For this review, use the dimensioned drawing (mm, ordinates from the lowest corner) and the shaded views. A direction names the side the tool comes from. Coordinates: 2 decimals unless noted, no trailing zeros. Loops run counter-clockwise (first coordinate to the right, second up) from the corner with the lowest first, then second, coordinate; pieces in that order, holes last. Notation, with made-up numbers: (15.25, 73.25) - (47.25, 73.25) arc R21 ccw to (47.25, 81.25) - close; hole circle Ø1 at (-30.5, -13). An arc over 180 degrees is marked (long way). Use a Markdown table: item, result. Add a question column.
1) The part is to be moulded in two halves that separate along Y. For the marked faces 1, 2 and 3, say which applies: pulls with the +Y half, pulls with the -Y half, needs draft (parallel to the pull), parting line crosses it, or undercut.
2) Add section C-C, the plane y = 45. Give the boundary of the cut face in (x, z), and give its area (3 significant figures).
3) Add section A-A, the plane z = 18. Give the boundary of the cut face in (x, y), and give its area (3 significant figures).
4) Add section D-D, the plane x = 43.5. Give the boundary of the cut face in (y, z), and give its area (3 significant figures).
5) For the marked faces 4 and 5, list the 3-axis set-ups (+Z, -Z, +X, -X, +Y, -Y) from which the entire face can be reached by the end or side of a thin tool; tool diameter is ignored.
6) Add section B-B, the plane x = 130. Give the boundary of the cut face in (y, z).
7) Clearance check with flat-ended pins moving along their axes: pin 1 (19 mm diameter, centred on x = 44.5, y = 32, fed in from -Z); pin 2 (6 mm diameter, centred on x = 19.5, z = 35, fed in from +Y). State where each tip first meets the part, or that it passes through.
8) To check wall thickness, follow L1, parallel to Y at x = 86.5, z = 7; L2, parallel to Z at x = 14.5, y = 57; L3, parallel to Y at x = 130, z = 35. State the ranges of each line that lie inside material, in increasing order. Write a range as [from, to].
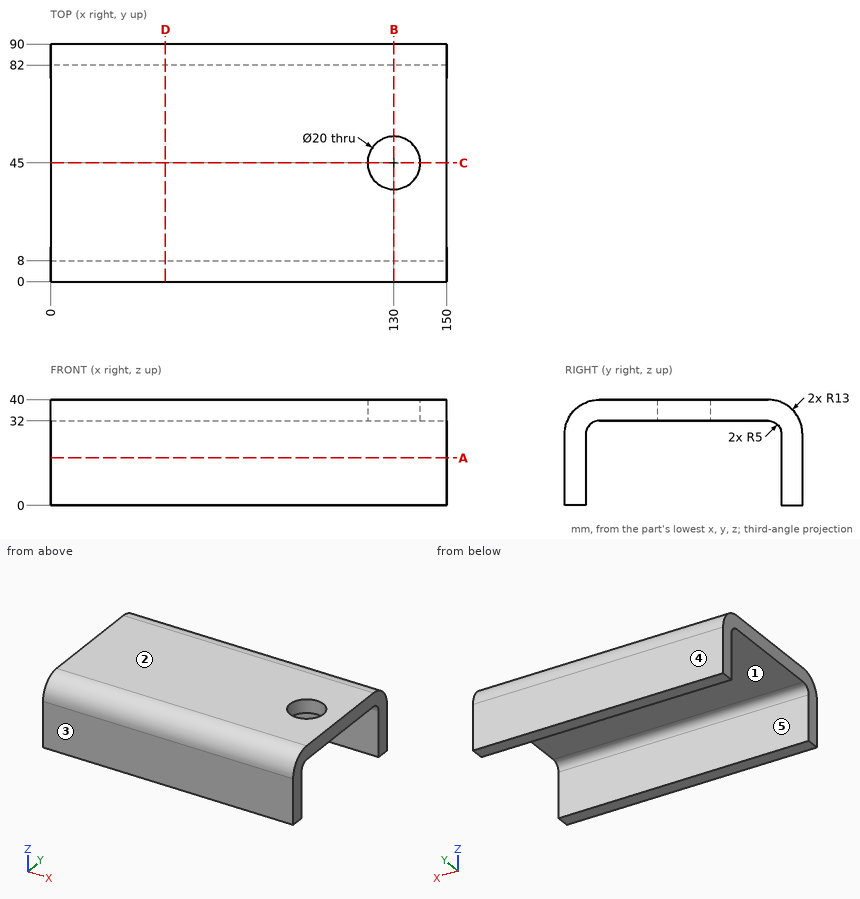
From the geometry:
| question | item | result |
|---|---|---|
| 1 | face 1 | undercut |
| 1 | face 2 | needs draft |
| 1 | face 3 | pulls with the -Y half |
| 2 | outline | (0, 32) - (120, 32) - (120, 40) - (0, 40) - close; (140, 32) - (150, 32) - (150, 40) - (140, 40) - close |
| 2 | area | 1,040 mm^2 |
| 3 | outline | (0, 0) - (150, 0) - (150, 8) - (0, 8) - close; (0, 82) - (150, 82) - (150, 90) - (0, 90) - close |
| 3 | area | 2,400 mm^2 |
| 4 | outline | (0, 0) - (8, 0) - (8, 27) arc R5 cw to (13, 32) - (77, 32) arc R5 cw to (82, 27) - (82, 0) - (90, 0) - (90, 27) arc R13 ccw to (77, 40) - (13, 40) arc R13 ccw to (0, 27) - close |
| 4 | area | 1,170 mm^2 |
| 5 | face 4 | +Z, -Z, +X, -X, +Y |
| 5 | face 5 | -Z, +X, -X |
| 6 | outline | (0, 0) - (8, 0) - (8, 27) arc R5 cw to (13, 32) - (35, 32) - (35, 40) - (13, 40) arc R13 ccw to (0, 27) - close; (55, 32) - (77, 32) arc R5 cw to (82, 27) - (82, 0) - (90, 0) - (90, 27) arc R13 ccw to (77, 40) - (55, 40) - close |
| 7 | pin 1 | stops at z = 32 |
| 7 | pin 2 | stops at y = 89 |
| 8 | L1 | y = [0, 8], [82, 90] |
| 8 | L2 | z = [32, 40] |
| 8 | L3 | y = [2.75, 35], [55, 87.25] |
